Input: part model. Units: mm. Frame: model coordinates. Coordinates: 2 decimals unless noted, no trailing zeros. Write each loop counter-clockwise with the first axis right and the second up, starting at its lowest first coordinate (ties: lowest second). Pieces come first, ordered by that corner, then holes. Notation, with made-up numbers: (-24.75, 26.25) - (9.25, 26.25) arc R28 cw to (9.25, 61.25) - close; hole circle Ø9 at (22, 38). An arc over 180 degrees is marked (long way). One line per question, with ' | ' between items. Start each with the question number.
1) Section query B-B on y = 12. Return loops of the section in (x, z), and give its area (3 significant figures).
2) Draft query along Y for faces 1 (the flat face through (35, 24, 12)), 2 (the cylindrical face through (5.63, 9.41, 12.17)), 3 (the flat face through (35, 12, 0)). Return one class per face: released by +Y, released by -Y, zero draft, split by the parting line, or undercut.
3) Section query A-A on x = 61. Return loops of the section in (y, z), and give its area (3 significant figures).
4) Line query: line 1 (Y direction, x = 61, z = 13.75); line 2 (X direction, y = 13.5, z = 21.5); line 3 (Y direction, x = 64.5, z = 8.5). Output: solid intervals per line, ascending.
5) Section query D-D on y = 15. Return loops of the section in (x, z).
6) Section query C-C on z = 7. Return loops of the section in (x, y), and give its area (3 significant figures).
```python
from build123d import *

# Parameters (mm, degrees)
SKETCH_1_W          = 70
SKETCH_1_H          = 24
EXTRUDE_1_DEPTH     = 24
SKETCH_2_R          = 4.25
CUT_EXTRUDE_1_DEPTH = 78.794601355


with BuildPart() as part:
    # 草图1 → 凸台-拉伸1 (new body)
    with BuildSketch(Plane.XY):
        with Locations((35, 12)):
            Rectangle(SKETCH_1_W, SKETCH_1_H)
    extrude(amount=EXTRUDE_1_DEPTH)

    # 草图2 → 切除-拉伸1 (cut, through all)
    with BuildSketch(Plane.XY.offset(24)):
        with Locations((9, 12)):
            Circle(SKETCH_2_R)
        with Locations(Location((61, 12, 0), (0, 0, 180))):
            Circle(SKETCH_2_R)
    extrude(amount=-CUT_EXTRUDE_1_DEPTH, mode=Mode.SUBTRACT)


solid = part.part
```
Answer key:
1) outline: (0, 0) - (4.75, 0) - (4.75, 24) - (0, 24) - close; (13.25, 0) - (56.75, 0) - (56.75, 24) - (13.25, 24) - close; (65.25, 0) - (70, 0) - (70, 24) - (65.25, 24) - close | area: 1,270 mm²
2) face 1: released by +Y | face 2: undercut | face 3: zero draft
3) outline: (0, 0) - (7.75, 0) - (7.75, 24) - (0, 24) - close; (16.25, 0) - (24, 0) - (24, 24) - (16.25, 24) - close | area: 372 mm²
4) line 1: 0 to 7.75, 16.25 to 24 | line 2: 0 to 5.02, 12.98 to 57.02, 64.98 to 70 | line 3: 0 to 9.59, 14.41 to 24
5) outline: (0, 0) - (5.99, 0) - (5.99, 24) - (0, 24) - close; (12.01, 0) - (57.99, 0) - (57.99, 24) - (12.01, 24) - close; (64.01, 0) - (70, 0) - (70, 24) - (64.01, 24) - close
6) outline: (0, 0) - (70, 0) - (70, 24) - (0, 24) - close; hole circle Ø8.5 at (9, 12); hole circle Ø8.5 at (61, 12) | area: 1,570 mm²
